```python
from build123d import *

# Parameters (mm, degrees)
SKETCH1_W            = 510
SKETCH1_H            = 80
BOSS_EXTRUDE1_DEPTH  = 10
SKETCH2_W            = 70
SKETCH2_H            = 390
CUT_EXTRUDE1_DEPTH   = 11
SKETCH3_W            = 70
SKETCH3_H            = 50
CUT_EXTRUDE2_DEPTH   = 11
SKETCH4_W            = 70
SKETCH4_H            = 10
BOSS_EXTRUDE2_DEPTH  = 100
SKETCH5_W            = 70
SKETCH5_H            = 50
CUT_EXTRUDE3_DEPTH   = 11
SKETCH6_W            = 70
SKETCH6_H            = 10
BOSS_EXTRUDE3_DEPTH  = 100
SKETCH7_W            = 10
SKETCH7_H            = 460
BOSS_EXTRUDE4_DEPTH  = 10
SKETCH8_W            = 10
SKETCH8_H            = 10
BOSS_EXTRUDE5_DEPTH  = 50
SKETCH9_W            = 90
SKETCH9_H            = 60
CUT_EXTRUDE4_DEPTH   = 61
SKETCH10_W           = 90
SKETCH10_H           = 60
CUT_EXTRUDE5_DEPTH   = 61
HOLE1_D              = 6.35
HOLE1_DEPTH          = 10
HOLE2_D              = 6.35
HOLE2_DEPTH          = 80
SCALE1_SCALE         = 4
SKETCH16_W           = 420.354500644
SKETCH16_H           = 2047.440969125
SKETCH16_W_2         = 504.269615058
SKETCH16_H_2         = 2143.883100275
CUT_EXTRUDE6_DEPTH   = 600
SKETCH17_W           = 706.747089412
SKETCH17_H           = 1090.886123918
CUT_EXTRUDE7_DEPTH   = 100
SKETCH18_W           = 40
SKETCH18_H           = 25
BOSS_EXTRUDE6_DEPTH  = 1
SKETCH20_W           = 40
SKETCH20_H           = 1219
SKETCH20_R           = 12.7
BOSS_EXTRUDE9_DEPTH  = 25
SKETCH21_W           = 440
SKETCH21_H           = 40
BOSS_EXTRUDE10_DEPTH = 25


with BuildPart() as part:
    # Sketch1 → Boss-Extrude1 (new body)
    with BuildSketch(Plane(origin=(45, 0, 0), x_dir=(0, -1, 0), z_dir=(-1, 0, 0))):
        with Locations((217.383525535, 40)):
            Rectangle(SKETCH1_W, SKETCH1_H)
    extrude(amount=-BOSS_EXTRUDE1_DEPTH)

    # Sketch2 → Cut-Extrude1 (cut, through all)
    with BuildSketch(Plane.ZY.offset(-45)):
        with Locations((35, -217.383525535)):
            Rectangle(SKETCH2_W, SKETCH2_H)
    extrude(amount=-CUT_EXTRUDE1_DEPTH, mode=Mode.SUBTRACT)

    # Sketch3 → Cut-Extrude2 (cut, through all)
    with BuildSketch(Plane.ZY.offset(-45)):
        with Locations((35, 12.616474465)):
            Rectangle(SKETCH3_W, SKETCH3_H)
    extrude(amount=-CUT_EXTRUDE2_DEPTH, mode=Mode.SUBTRACT)

    # Sketch4 → Boss-Extrude2 (add)
    with BuildSketch(Plane.ZY.offset(-45)):
        with Locations((35, -17.383525535)):
            Rectangle(SKETCH4_W, SKETCH4_H)
    extrude(amount=BOSS_EXTRUDE2_DEPTH)

    # Sketch5 → Cut-Extrude3 (cut, through all)
    with BuildSketch(Plane.ZY.offset(-45)):
        with Locations((35, -447.383525535)):
            Rectangle(SKETCH5_W, SKETCH5_H)
    extrude(amount=-CUT_EXTRUDE3_DEPTH, mode=Mode.SUBTRACT)

    # Sketch6 → Boss-Extrude3 (add)
    with BuildSketch(Plane.ZY.offset(-45)):
        with Locations((35, -417.383525535)):
            Rectangle(SKETCH6_W, SKETCH6_H)
    extrude(amount=BOSS_EXTRUDE3_DEPTH)

    # Sketch7 → Boss-Extrude4 (add)
    with BuildSketch(Plane.XY.offset(70)):
        with Locations((-50, -242.383525535)):
            Rectangle(SKETCH7_W, SKETCH7_H)
    extrude(amount=BOSS_EXTRUDE4_DEPTH)

    # Sketch8 → Boss-Extrude5 (add)
    with BuildSketch(Plane(origin=(0, -12.383525535, 0), x_dir=(-1, 0, 0), z_dir=(0, 1, 0))):
        with Locations((50, 75)):
            Rectangle(SKETCH8_W, SKETCH8_H)
    extrude(amount=BOSS_EXTRUDE5_DEPTH)

    # Sketch9 → Cut-Extrude4 (cut, through all)
    with BuildSketch(Plane.XZ.offset(22.383525535)):
        with Locations((0, 30)):
            Rectangle(SKETCH9_W, SKETCH9_H)
    extrude(amount=-CUT_EXTRUDE4_DEPTH, mode=Mode.SUBTRACT)

    # Sketch10 → Cut-Extrude5 (cut, through all)
    with BuildSketch(Plane(origin=(0, -412.383525535, 0), x_dir=(-1, 0, 0), z_dir=(0, 1, 0))):
        with Locations((0, 30)):
            Rectangle(SKETCH10_W, SKETCH10_H)
    extrude(amount=-CUT_EXTRUDE5_DEPTH, mode=Mode.SUBTRACT)

    # Hole1
    with Locations(Plane(origin=(0, 0, 70), x_dir=(-1, 0, 0), z_dir=(0, 0, -1))):
        with Locations((-50, 27.616474465), (50, -462.383525535)):
            Hole(HOLE1_D / 2, depth=HOLE1_DEPTH)

    # Hole2
    with Locations(Plane.XY.offset(80)):
        with Locations((50, -462.383525535), (-50, 27.616474465)):
            Hole(HOLE2_D / 2, depth=HOLE2_DEPTH)


with BuildPart() as part_1:
    # Scale1: scaled about (0, -217.383525535, 66.140384571)
    add(part.part.scale(SCALE1_SCALE).moved(Location((0, 652.150576605, -198.421153713))))

    # Sketch16 → Cut-Extrude6 (cut)
    with BuildSketch(Plane(origin=(220, 0, 0), x_dir=(0, 0, -1), z_dir=(1, 0, 0))):
        with Locations((153.598404035, -157.332882586)):
            Rectangle(SKETCH16_W, SKETCH16_H)
        with Locations((-358.713653816, -248.900281802)):
            Rectangle(SKETCH16_W_2, SKETCH16_H_2)
    extrude(amount=-CUT_EXTRUDE6_DEPTH, mode=Mode.SUBTRACT)

    # Sketch17 → Cut-Extrude7 (cut)
    with BuildSketch(Plane.XY.offset(106.578846287)):
        with Locations((133.373544706, 328.059536424)):
            Rectangle(SKETCH17_W, SKETCH17_H)
    extrude(amount=-CUT_EXTRUDE7_DEPTH, mode=Mode.SUBTRACT)

    # Sketch18 → Boss-Extrude6 (add)
    with BuildSketch(Plane(origin=(0, -217.383525535, 0), x_dir=(1, 0, 0), z_dir=(0, 1, 0))):
        with Locations((-200, -94.078846287)):
            Rectangle(SKETCH18_W, SKETCH18_H)
        with Locations((200, -94.078846287)):
            Rectangle(SKETCH18_W, SKETCH18_H)
    extrude(amount=BOSS_EXTRUDE6_DEPTH)

    # Sketch20 → Boss-Extrude9 (add)
    with BuildSketch(Plane.XY.offset(106.578846287)):
        with Locations((-200, 393.116474465)):
            Rectangle(SKETCH20_W, SKETCH20_H)
        with Locations((-200, 962.616474465)):
            Circle(SKETCH20_R, mode=Mode.SUBTRACT)
        with Locations((200, 393.116474465)):
            Rectangle(SKETCH20_W, SKETCH20_H)
        with Locations((200, 962.616474465)):
            Circle(SKETCH20_R, mode=Mode.SUBTRACT)
    extrude(amount=-BOSS_EXTRUDE9_DEPTH)

    # Sketch21 → Boss-Extrude10 (add)
    with BuildSketch(Plane(origin=(0, 0, 81.578846287), x_dir=(-1, 0, 0), z_dir=(0, 0, -1))):
        with Locations((0, 782.616474465)):
            Rectangle(SKETCH21_W, SKETCH21_H)
    extrude(amount=BOSS_EXTRUDE10_DEPTH)


solid = part_1.part
```
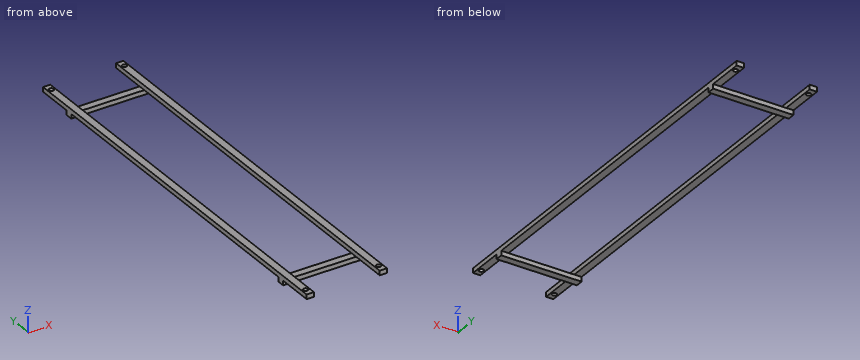
Input: part model. Units: mm. Frame: model coordinates. Give positions to 0.01 mm unless a question says otherwise; leave off trailing zeros. Order: outer loops, then holes, each group sorted by start corner. A loop starts at its lowest first (then second) coordinate and runs counter-clockwise, first axis right, second up. Notation, with made-up numbers: M 49,-21 L 93,-21 A26 ccw 93,1 Z; hole C 74.25,47 d11. An arc over 180 degrees is marked long. One line per question, with ' | ' between items. Start each with the question number.
1. Section query A-A (z = 67). Return the cut outline in (x, y).
2. Material intervals for probe 1 along X at (y, z) = (-564.5, 99); probe 2 along Y at (x, z) = (142, 74); probe 3 along Z at (x, y) = (-190, -908.5), sorted ascending. Write a range as [from, to].
3. First-contact query: pin 1 Ø12 at (x, y) = (57.5, 773.5) entering from +Z; pin 2 Ø7.5 at (x, z) = (93, 74) entering from -Y; pin 3 Ø20 at (x, y) = (192, -257) entering from -Z. Flat tips, straight axial feed; report the tip coordinate or a pass-through.
4. Section query B-B (y = -359). Return the cut outline in (x, z).
Here are the results:
1) outline: M -220,-1037.38 L 220,-1037.38 L 220,-997.38 L -220,-997.38 Z; M -220,762.62 L 220,762.62 L 220,802.62 L -220,802.62 Z
2) probe 1: [-220, -180], [180, 220] | probe 2: [-1037.38, -997.38], [762.62, 802.62] | probe 3: [81.58, 106.58]
3) pin 1: z = 81.58 | pin 2: y = -1037.38 | pin 3: z = 81.58
4) outline: M -220,81.58 L -180,81.58 L -180,106.58 L -220,106.58 Z; M 180,81.58 L 220,81.58 L 220,106.58 L 180,106.58 Z
